Build history of the part. All positions in model axes, mm. A direction names the side the tool comes from. Give positions to 0.01 mm unless a question says otherwise; leave off trailing zeros. Write each loop counter-clockwise with the first axis right and the second up, starting at its lowest first coordinate (ties: lowest second). Pieces come first, ordered by that corner, then holes. Notation, with made-up numbers: M -14,-40 L 8,-40 A36 cw 8,-3 Z; hole C 66,11 d2. An arc over 180 degrees is marked long. One line per item, written item: value. Start each with the question number.
from build123d import *

# Parameters (mm, degrees)
ESQUISSE1_R                  = 61.25
ESQUISSE1_R_2                = 41.25
BOSS_EXTRU_1_DEPTH           = 15
ENL_V_MAT_EXTRU_1_DEPTH      = 88.909754863
ENL_V_MAT_EXTRU_1_DEPTH_BACK = 88.909754863
ENL_V_MAT_EXTRU_2_DEPTH      = 88.909754863
ENL_V_MAT_EXTRU_2_DEPTH_BACK = 88.909754863
CONG_1_R                     = 2
CONG_2_R                     = 3
ENL_V_MAT_EXTRU_3_DEPTH      = 88.909754863
ENL_V_MAT_EXTRU_3_DEPTH_BACK = 88.909754863
ESQUISSE4_R                  = 2.5


with BuildPart() as part:
    # Esquisse1 → Boss.-Extru.1 (new body)
    with BuildSketch(Plane.XY):
        Circle(ESQUISSE1_R)
        Circle(ESQUISSE1_R_2, mode=Mode.SUBTRACT)
    extrude(amount=BOSS_EXTRU_1_DEPTH)

    # Esquisse2 → Enlèv. mat.-Extru.1 (cut, two sides: drawn at the far end of the back side and taken through both)
    with BuildSketch(Plane.XY.offset(15).offset(-ENL_V_MAT_EXTRU_1_DEPTH_BACK)):
        Polygon((26.395724667, 31.699025526), (31.699025526, 26.395724667), (37.002326385, 31.699025526), (31.699025526, 37.002326385), align=None)
        Polygon((31.699025526, -26.395724667), (26.395724667, -31.699025526), (31.699025526, -37.002326385), (37.002326385, -31.699025526), align=None)
        Polygon((-26.395724667, -31.699025526), (-31.699025526, -26.395724667), (-37.002326385, -31.699025526), (-31.699025526, -37.002326385), align=None)
        Polygon((-31.699025526, 26.395724667), (-26.395724667, 31.699025526), (-31.699025526, 37.002326385), (-37.002326385, 31.699025526), align=None)
    extrude(amount=ENL_V_MAT_EXTRU_1_DEPTH + ENL_V_MAT_EXTRU_1_DEPTH_BACK, mode=Mode.SUBTRACT)

    # Esquisse3 → Enlèv. mat.-Extru.2 (cut, two sides: drawn at the far end of the back side and taken through both)
    with BuildSketch(Plane.XY.offset(15).offset(-ENL_V_MAT_EXTRU_2_DEPTH_BACK)):
        with BuildLine():
            Line((-26.727272727, -55.110937141), (-18, -37.115529095))
            ThreePointArc((-18, -37.115529095), (0, -41.25), (18, -37.115529095))
            Line((18, -37.115529095), (26.727272727, -55.110937141))
            ThreePointArc((26.727272727, -55.110937141), (0, -61.25), (-26.727272727, -55.110937141))
        make_face()
    extrude(amount=ENL_V_MAT_EXTRU_2_DEPTH + ENL_V_MAT_EXTRU_2_DEPTH_BACK, mode=Mode.SUBTRACT)

    # Congé1
    cong_1_edges = [part.edges().sort_by_distance(p)[0] for p in [
        (-31.699025526, 37.002326385, 7.5),
        (-26.395724667, 31.699025526, 7.5),
        (-31.699025526, 26.395724667, 7.5),
        (-37.002326385, 31.699025526, 7.5),
        (-37.002326385, -31.699025526, 7.5),
        (-31.699025526, -26.395724667, 7.5),
        (-26.395724667, -31.699025526, 7.5),
        (-31.699025526, -37.002326385, 7.5),
        (31.699025526, -37.002326385, 7.5),
        (26.395724667, -31.699025526, 7.5),
        (31.699025526, -26.395724667, 7.5),
        (37.002326385, -31.699025526, 7.5),
        (37.002326385, 31.699025526, 7.5),
        (31.699025526, 26.395724667, 7.5),
        (26.395724667, 31.699025526, 7.5),
        (31.699025526, 37.002326385, 7.5),
    ]]
    fillet(cong_1_edges, radius=CONG_1_R)

    # Congé2
    cong_2_edges = [part.edges().sort_by_distance(p)[0] for p in [
        (-18, -37.115529095, 7.5),
        (18, -37.115529095, 7.5),
        (26.727272727, -55.110937141, 7.5),
        (-26.727272727, -55.110937141, 7.5),
    ]]
    fillet(cong_2_edges, radius=CONG_2_R)

    # Esquisse4 → Enlèv. mat.-Extru.3 (cut, two sides: drawn at the far end of the back side and taken through both)
    with BuildSketch(Plane.XY.offset(15).offset(-ENL_V_MAT_EXTRU_3_DEPTH_BACK)):
        with Locations((-30, -45)):
            Circle(ESQUISSE4_R)
        with Locations((30, -45)):
            Circle(ESQUISSE4_R)
        with Locations((-47.92432366, -17.44302731)):
            Circle(ESQUISSE4_R)
        with Locations((-25.5, 44.167295593)):
            Circle(ESQUISSE4_R)
        with Locations((25.5, 44.167295593)):
            Circle(ESQUISSE4_R)
        with Locations((47.92432366, -17.44302731)):
            Circle(ESQUISSE4_R)
    extrude(amount=ENL_V_MAT_EXTRU_3_DEPTH + ENL_V_MAT_EXTRU_3_DEPTH_BACK, mode=Mode.SUBTRACT)


solid = part.part
1) Tool access for faces 3 (the face through (22.28, -45.94, 7.39)), 4 (the face through (31.721, -36.174, 7.605)): list every direction of +Z, -Z, +X, -X, +Y, -Y with a clear straight run to the whole face (end or side of a thin tool).
2) Band-saw the part on A-A (y = 0). List the corners of the cut face in (x, z).
3) Mould opens along X. For faces 1 (the face through (-1, 43, 15)), 2 (the face through (50.234, -18.401, 7.395)) say: released by +X, released by -X, zero draft, split by the parting line, or undercut.
4) Band-saw the part on B-B (y = -45). List the corners of the cut face in (x, z), then the cut area to 3 significant figures.
5) Drop flat-ended pins along their axis: P1, Ø6, axis at x = 21, z = 2.5, coming from the -Y side; P2, Ø8, axis at x = -43.5, z = 5, coming from the +Y side; P3, Ø6, axis at y = -21, z = 7, coming from the -X side. Give the stop position or say it passes through.
6) Probe line 1 along Y through (x, z) = (-30, 6.75); line 2 along Y through (x, z) = (24, 9.25); line 3 along Y through (x, z) = (-34.5, 12). List the from-to ranges inside material, lowest first. Write a range as from..to.
7) Band-saw the part on D-D (z = 8.5). Count the separate pieces of the cut face and the enclosed holes in it, then the cut area to 3 significant figures.
8) Band-saw the part on C-C (x = 0). List the corners of the cut face in (y, z), then the cut area to 3 significant figures.
Model answer:
1. face 3: +Z, -Z, -Y
1. face 4: +Z, -Z
2. outline: M -61.25,0 L -41.25,0 L -41.25,15 L -61.25,15 Z; M 41.25,0 L 61.25,0 L 61.25,15 L 41.25,15 Z
3. face 1: zero draft
3. face 2: undercut
4. outline: M -41.55,0 L -32.5,0 L -32.5,15 L -41.55,15 Z; M -27.5,0 L -21.82,0 L -21.82,15 L -27.5,15 Z; M 21.82,0 L 27.5,0 L 27.5,15 L 21.82,15 Z; M 32.5,0 L 41.55,0 L 41.55,15 L 32.5,15 Z
4. area: 442 mm²
5. P1: stops at y = -49.49
5. P2: stops at y = 46.81
5. P3: stops at x = -58.55
6. line 1: y = -53.4..-47.5, -42.5..-35.3, 35.3..53.4
6. line 2: y = -49.49..-33.55, 33.55..42.17, 46.17..56.35
6. line 3: y = -50.61..-34.2, -29.2..-22.61, 22.61..29.2, 34.2..50.61
7. separate pieces: 1
7. enclosed holes: 6
7. area: 5,170 mm²
8. outline: M 41.25,0 L 61.25,0 L 61.25,15 L 41.25,15 Z
8. area: 300 mm²
